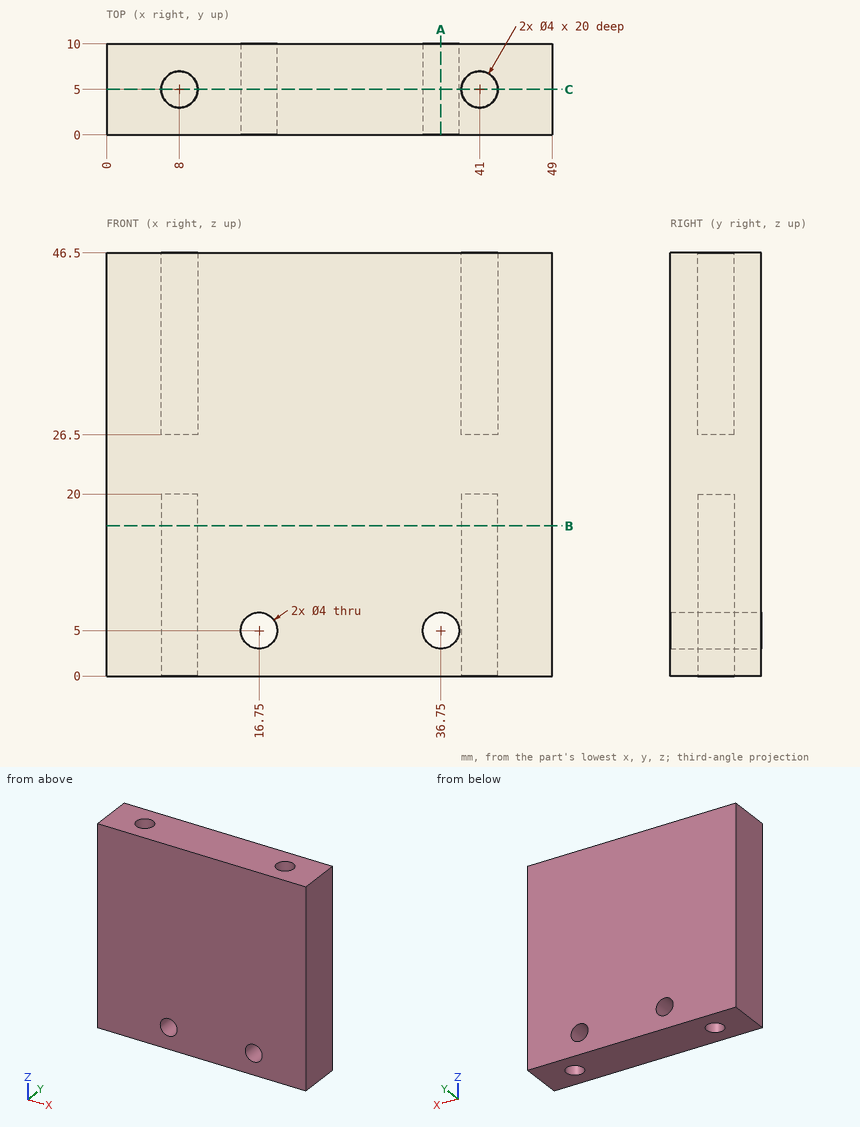
Verification items for this drawing (mm, ordinates from the low corner). Coordinates: 2 decimals unless noted, no trailing zeros. Write each loop counter-clockwise with the first axis right and the second up, starting at its lowest first coordinate (ties: lowest second). Pieces come first, ordered by that corner, then holes. Notation, with made-up numbers: M 48,-4 L 91,-4 A18 ccw 91,2 Z; hole C -0.75,54 d6. An arc over 180 degrees is marked long. Answer as CSV lines item,"result".
Q1. Cross-section at A-A (x = 36.75). Record the boundary of the cut face in (y, z), then the cut area to 3 significant figures.
Check result:
outline,"M 0,0 L 10,0 L 10,3 L 0,3 Z; M 0,7 L 10,7 L 10,46.5 L 0,46.5 Z"
area,"425 mm^2"
Q2. Cross-section at C-C (y = 5). Record the boundary of the cut face in (x, z).
Check result:
outline,"M 0,0 L 6,0 L 6,20 L 10,20 L 10,0 L 39,0 L 39,20 L 43,20 L 43,0 L 49,0 L 49,46.5 L 43,46.5 L 43,26.5 L 39,26.5 L 39,46.5 L 10,46.5 L 10,26.5 L 6,26.5 L 6,46.5 L 0,46.5 Z; hole C 16.75,5 d4; hole C 36.75,5 d4"
Q3. Material ranges on probe 1 along X at (y, z) = (5, 12.25); probe 2 along Z at (x, y) = (16.75, 4); probe 3 along X at (y, z) = (6, 2), recorded low to high. Write a range as from..to.
Check result:
probe 1,"0..6, 10..39, 43..49"
probe 2,"0..3, 7..46.5"
probe 3,"0..6.27, 9.73..39.27, 42.73..49"
Q4. Go/stop test with flat-tipped pins: pin 1 (3.5 mm diameter, centred on x = 41, y = 5, fed in from +Z); pin 2 (3.5 mm diameter, centred on x = 16.75, z = 5, fed in from -Y); pin 3 (3 mm diameter, centred on x = 19.5, y = 1, fed in from -Z); pin 4 (3.5 mm diameter, centred on x = 41, y = 5, fed in from -Z). Record where each tip stops, or that it passes through.
Check result:
pin 1,"z = 26.5"
pin 2,"through"
pin 3,"z = 0"
pin 4,"z = 20"
Q5. Cross-section at B-B (z = 16.5). Record the boundary of the cut face in (x, y), then the cut area to 3 significant figures.
Check result:
outline,"M 0,0 L 49,0 L 49,10 L 0,10 Z; hole C 8,5 d4; hole C 41,5 d4"
area,"465 mm^2"
